from build123d import *

# Parameters (mm, degrees)
SKETCH_1_W          = 44
SKETCH_1_H          = 76
SKETCH_1_W_2        = 40
SKETCH_1_H_2        = 72
EXTRUDE_1_DEPTH     = 50
SKETCH_2_R          = 2.15
CUT_EXTRUDE_1_DEPTH = 102.054440773
CUT_EXTRUDE_2_REACH = 103.054
SKETCH_3_R          = 17.525
CUT_EXTRUDE_3_REACH = 103.054
SKETCH_4_R          = 10.525
SKETCH_12_R         = 2
CUT_EXTRUDE_7_DEPTH = 10


with BuildPart() as part:
    # 草图1 → 凸台-拉伸1 (new body)
    with BuildSketch(Plane(origin=(0, 0, 0), x_dir=(1, 0, 0), z_dir=(0, 1, 0))):
        with Locations((22, -38)):
            Rectangle(SKETCH_1_W, SKETCH_1_H)
        with Locations((22, -38)):
            Rectangle(SKETCH_1_W_2, SKETCH_1_H_2, mode=Mode.SUBTRACT)
    extrude(amount=EXTRUDE_1_DEPTH)

    # 草图2 → 切除-拉伸1 (cut, through all)
    with BuildSketch(Plane(origin=(0, 0, 0), x_dir=(-1, 0, 0), z_dir=(0, 0, -1))):
        with Locations((-10.5, 6.5)):
            Circle(SKETCH_2_R)
        with Locations((-37.5, 6.5)):
            Circle(SKETCH_2_R)
        with Locations((-37.5, 43.5)):
            Circle(SKETCH_2_R)
        with Locations((-10.5, 43.5)):
            Circle(SKETCH_2_R)
    extrude(amount=-CUT_EXTRUDE_1_DEPTH, mode=Mode.SUBTRACT)

    # 草图3 → Cut-Extrude 2 (cut, up to next)
    with BuildSketch(Plane.ZY, mode=Mode.PRIVATE) as cut_extrude_2_sk1:
        with Locations((25, 25)):
            Circle(SKETCH_3_R)
    cut_extrude_2_tool1 = extrude(cut_extrude_2_sk1.sketch, amount=-CUT_EXTRUDE_2_REACH, mode=Mode.PRIVATE) & part.part
    add(cut_extrude_2_tool1.solids().sort_by_distance((0, 25, 25))[0], mode=Mode.SUBTRACT)

    # 草图4 → Cut-Extrude 3 (cut, up to next)
    with BuildSketch(Plane(origin=(44, 0, 0), x_dir=(0, 0, -1), z_dir=(1, 0, 0)), mode=Mode.PRIVATE) as cut_extrude_3_sk1:
        with Locations((-25, 25)):
            Circle(SKETCH_4_R)
    cut_extrude_3_tool1 = extrude(cut_extrude_3_sk1.sketch, amount=-CUT_EXTRUDE_3_REACH, mode=Mode.PRIVATE) & part.part
    add(cut_extrude_3_tool1.solids().sort_by_distance((44, 25, 25))[0], mode=Mode.SUBTRACT)

    # 草图12 → 电机7号 (cut)
    with BuildSketch(Plane(origin=(44, 0, 0), x_dir=(0, 0, -1), z_dir=(1, 0, 0))):
        with Locations((-12.303937618, 30.9)):
            Circle(SKETCH_12_R)
        with Locations((-19.1, 12.303937618)):
            Circle(SKETCH_12_R)
        with Locations((-37.696062382, 19.1)):
            Circle(SKETCH_12_R)
        with Locations((-30.9, 37.696062382)):
            Circle(SKETCH_12_R)
    extrude(amount=-CUT_EXTRUDE_7_DEPTH, mode=Mode.SUBTRACT)


solid = part.part
Can you work these out from the model? Positions are in its coordinate system, mm. A direction names the side the tool comes from. Give positions to 0.01 mm unless a question says otherwise; leave off trailing zeros. Write each loop counter-clockwise with the first axis right and the second up, starting at its lowest first coordinate (ties: lowest second). Pieces come first, ordered by that corner, then holes. Notation, with made-up numbers: M -39.5,69 L 0.5,69 A26 ccw 0.5,105 Z; hole C 9.5,-3.5 d6. An arc over 180 degrees is marked long. Answer in a Markdown table with one row per item. Add a question column.
Item 1: Imagine slicing it at D-D, the plane y = 26. Write out the boundary of the cut face in (x, z), plus the area to 3 significant figures.
Item 2: On a 3-axis mill with a long thin cutter (end or side, diameter ignored), from which of +Z, -Z, +X, -X, +Y, -Y can I reach the whole of each face in a straight line? I mean faces 1 (the cylindrical face through (0.99, 14.34, 11.09)), 2 (the flat face through (22, 25, 74)), 3 (the cylindrical face through (43.01, 28.95, 12.74)). Say none if no direction works.
Item 3: We'd pull the mould along Z, two halves only. Please class faces 4 (the flat face through (22, 25, 76)), 5 (the cylindrical face through (43.01, 35.92, 29.98)), 6 (the cylindrical face through (43.014, 33.875, 19.342)), 7 (the cylindrical face through (9.34, 45.31, 0.99)): released by +Z, released by -Z, zero draft, split by the parting line, or undercut.
Item 4: Please list where these lines run through material, in increasing order: L1, parallel to Z at x = 3.5, y = 17; L2, parallel to X at y = 10.5, z = 40; L3, parallel to Y at x = 37.5, z = 0.6.
Item 5: Imagine slicing it at A-A, the plane x = 23. Write out the boundary of the cut face in (y, z).
Item 6: For pin 1 Ø3.5 at (y, z) = (30.9, 12.3) entering from +X; pin 2 Ø5 at (x, y) = (37.5, 43.5) entering from +Z; pin 3 Ø5 at (y, z) = (19.1, 37.7) entering from -X, each with a flat end and sliding along its axis, tell me the tip position at first contact or that it passes through.
Item 7: Imagine slicing it at B-B, the plane x = 10.5. Write out the boundary of the cut face in (y, z), plus the area to 3 significant figures.
Item 8: Imagine slicing it at C-C, the plane z = 25. Write out the boundary of the cut face in (x, y) (3 decimals), plus the area to 3 significant figures.
Evaluation:
| question | item | result |
|---|---|---|
| 1 | outline | M 0,0 L 44,0 L 44,14.52 L 42,14.52 L 42,2 L 2,2 L 2,7.5 L 0,7.5 Z; M 0,42.5 L 2,42.5 L 2,74 L 42,74 L 42,35.48 L 44,35.48 L 44,76 L 0,76 Z |
| 1 | area | 352 mm² |
| 2 | face 1 | -X |
| 2 | face 2 | +Y, -Y |
| 2 | face 3 | +X, -X |
| 3 | face 4 | released by +Z |
| 3 | face 5 | undercut |
| 3 | face 6 | undercut |
| 3 | face 7 | zero draft |
| 4 | L1 | z = 0 to 2, 74 to 76 |
| 4 | L2 | x = 0 to 2, 42 to 44 |
| 4 | L3 | y = 0 to 4.35, 8.65 to 41.35, 45.65 to 50 |
| 5 | outline | M 0,0 L 50,0 L 50,2 L 0,2 Z; M 0,74 L 50,74 L 50,76 L 0,76 Z |
| 6 | pin 1 | passes through |
| 6 | pin 2 | stops at z = 76 |
| 6 | pin 3 | stops at x = 42 |
| 7 | outline | M 0,0 L 4.35,0 L 4.35,2 L 0,2 Z; M 0,74 L 4.35,74 L 4.35,76 L 0,76 Z; M 8.65,0 L 41.35,0 L 41.35,2 L 8.65,2 Z; M 8.65,74 L 41.35,74 L 41.35,76 L 8.65,76 Z; M 45.65,0 L 50,0 L 50,2 L 45.65,2 Z; M 45.65,74 L 50,74 L 50,76 L 45.65,76 Z |
| 7 | area | 166 mm² |
| 8 | outline | M 0,0 L 2,0 L 2,7.475 L 0,7.475 Z; M 0,42.525 L 2,42.525 L 2,50 L 0,50 Z; M 42,0 L 44,0 L 44,14.475 L 42,14.475 Z; M 42,35.525 L 44,35.525 L 44,50 L 42,50 Z |
| 8 | area | 87.8 mm² |
